from build123d import *

# Parameters (mm, degrees)
SKETCH_1_W          = 135
SKETCH_1_H          = 145
EXTRUDE_1_DEPTH     = 90
SKETCH_2_W          = 130
SKETCH_2_H          = 140
CUT_EXTRUDE_1_DEPTH = 85
SKETCH_3_W          = 69
SKETCH_3_H          = 112
CUT_EXTRUDE_2_DEPTH = 5
SKETCH_4_R          = 1.4
CUT_EXTRUDE_3_DEPTH = 5
FILLET_1_R          = 10


with BuildPart() as part:
    # 草图1 → 凸台-拉伸1 (new body)
    with BuildSketch(Plane(origin=(0, 0, 0), x_dir=(1, 0, 0), z_dir=(0, 1, 0))):
        with Locations((67.5, -72.5)):
            Rectangle(SKETCH_1_W, SKETCH_1_H)
    extrude(amount=EXTRUDE_1_DEPTH)

    # 草图2 → 切除-拉伸1 (cut)
    with BuildSketch(Plane(origin=(0, 90, 0), x_dir=(1, 0, 0), z_dir=(0, 1, 0))):
        with Locations((65, -75)):
            Rectangle(SKETCH_2_W, SKETCH_2_H)
    extrude(amount=-CUT_EXTRUDE_1_DEPTH, mode=Mode.SUBTRACT)

    # 草图3 → 切除-拉伸2 (cut)
    with BuildSketch(Plane(origin=(0, 5, 0), x_dir=(1, 0, 0), z_dir=(0, 1, 0))):
        with Locations((34.5, -89)):
            Rectangle(SKETCH_3_W, SKETCH_3_H)
    extrude(amount=-CUT_EXTRUDE_2_DEPTH, mode=Mode.SUBTRACT)

    # 草图4 → 切除-拉伸3 (cut)
    with BuildSketch(Plane(origin=(0, 5, 0), x_dir=(1, 0, 0), z_dir=(0, 1, 0))):
        with Locations(Location((64, -23, 0), (0, 0, 270))):
            Circle(SKETCH_4_R)
    extrude(amount=-CUT_EXTRUDE_3_DEPTH, mode=Mode.SUBTRACT)

    # 圆角1
    fillet_1_edges = [part.edges().sort_by_distance(p)[0] for p in [
        (130, 47.5, 5),
        (69, 2.5, 33),
        (135, 45, 0),
    ]]
    fillet(fillet_1_edges, radius=FILLET_1_R)


solid = part.part
Build history of the part. All positions in model axes, mm. A direction names the side the tool comes from. Give positions to 0.01 mm unless a question says otherwise; leave off trailing zeros. Loops run counter-clockwise (first coordinate to the right, second up) from the corner with the lowest first, then second, coordinate; pieces in that order, holes last. Notation, with made-up numbers: (-16, 62) - (22, 62) arc R6 cw to (22, 71) - close; hole circle Ø3 at (4, 33.25). An arc over 180 degrees is marked (long way). Write item = value, one per line. Start each with the question number.
1) Band-saw the part on A-A on x = 100. Give the cut face in (y, z).
2) Probe probe 1 along X at (y, z) = (2.55, 23); probe 2 along Y at (x, z) = (74, 106); probe 3 along X at (y, z) = (38, 57). List the from-to ranges inside material, lowest first. Write a range as from..to.
3) Band-saw the part on C-C on y = 26. Give the cut face in (x, z), plus the area to 4 significant figures.
4) Drop flat-ended pins along their axis: pin 1 Ø3.5 at (x, z) = (64, 23) entering from +Y; pin 2 Ø5.5 at (x, y) = (29.5, 3) entering from +Z; pin 3 Ø4 at (x, y) = (72.5, 71.5) entering from +Z. Give the stop position or say it passes through.
5) Tool access for faces 1 (the flat face through (69, 3, 95)), 2 (the flat face through (131, 25, 145)), 3 (the flat face through (130, 48, 81)): list every direction of +Z, -Z, +X, -X, +Y, -Y with a clear straight run to the whole face (end or side of a thin tool).
6) Band-saw the part on B-B on z = 31. Give the cut face in (x, y), plus the area to 3 significant figures.
Final values:
q1.outline = (0, 0) - (90, 0) - (90, 5) - (5, 5) - (5, 145) - (0, 145) - close
q2.probe_1 = 0..62.6, 65.4..135
q2.probe_2 = 0..5
q2.probe_3 = 130..135
q3.outline = (0, 0) - (125, 0) arc R10 ccw to (135, 10) - (135, 145) - (130, 145) - (130, 15) arc R10 cw to (120, 5) - (0, 5) - close
q3.area = 1,375 mm²
q4.pin_1 = 5
q4.pin_2 = 33
q4.pin_3 = 5
q5.face_1 = +Z, -X, +Y, -Y
q5.face_2 = +Z, +X, -X, +Y, -Y
q5.face_3 = +Z, -X, +Y
q6.outline = (0, 0) - (135, 0) - (135, 90) - (130, 90) - (130, 5) - (0, 5) - close
q6.area = 1,100 mm²
